Could you check a few things on this model? Use its own coordinates, in mm. Round coordinates to 2 decimals unless told otherwise and drop trailing zeros. Write each loop counter-clockwise with the first axis right and the second up, starting at its lowest first coordinate (ties: lowest second). Pieces come first, ordered by that corner, then holes. Notation, with made-up numbers: (26, 58) - (60, 58) arc R19 ccw to (60, 64) - close; hole circle Ø5 at (87, -27.5). An arc over 180 degrees is marked (long way). Put each result on its own line as item: value.
from build123d import *

# Parameters (mm, degrees)
F0_W     = 35
F0_H     = 35
F1_DEPTH = 35
F3_DEPTH = 35.001
F5_DEPTH = 35.001
F7_DEPTH = 35.001
F9_D     = 2.5
F11_D    = 2.5
F13_D    = 2.5


with BuildPart() as f1:
    # F0 (on Top) → F1 (new body)
    with BuildSketch(Plane.XY):
        with Locations((17.5, 17.5)):
            Rectangle(F0_W, F0_H)
    extrude(amount=F1_DEPTH)

    # F2 (on face) → F3 (cut, through all)
    with BuildSketch(Plane.XY.offset(35)):
        Polygon((35, 35), (0, 35), (35, 0), align=None)
    extrude(amount=-F3_DEPTH, mode=Mode.SUBTRACT)

    # F4 (on face) → F5 (cut, through all)
    with BuildSketch(Plane.XZ):
        Polygon((35, 35), (0, 0), (35, 0), align=None)
    extrude(amount=-F5_DEPTH, mode=Mode.SUBTRACT)

    # F6 (on face) → F7 (cut, through all)
    with BuildSketch(Plane(origin=(0, 0, 0), x_dir=(0, -1, 0), z_dir=(-1, 0, 0))):
        Polygon((-35, 0), (0, 0), (-35, 35), align=None)
    extrude(amount=-F7_DEPTH, mode=Mode.SUBTRACT)

    # F9 (through all)
    with Locations(Plane.XZ):
        with Locations((23, 30), (5, 12)):
            Hole(F9_D / 2)

    # F11 (through all)
    with Locations(Plane(origin=(0, 0, 0), x_dir=(0, -1, 0), z_dir=(-1, 0, 0))):
        with Locations((-23, 30), (-5, 12)):
            Hole(F11_D / 2)

    # F13 (through all)
    with Locations(Plane.XY.offset(35)):
        with Locations((5, 23), (23, 5)):
            Hole(F13_D / 2)


solid = f1.part
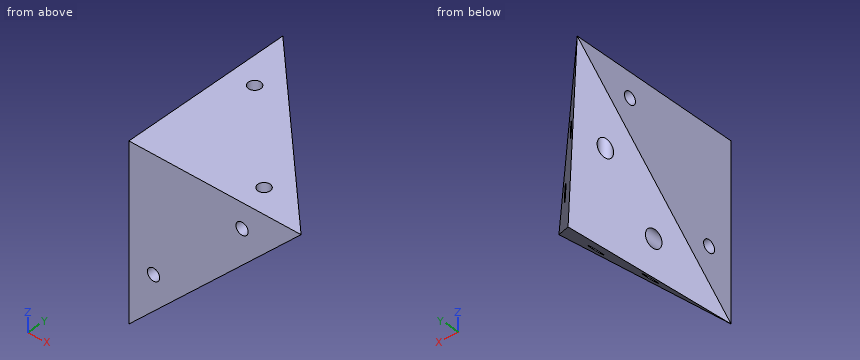
(1) Imagine slicing it at A-A, the plane y = 23. List the corners of the cut face in (x, z) for me.
Values found:
outline: (0, 23) - (3.75, 23) - (3.75, 28.75) - (0, 28.75) - close; (0, 31.25) - (3.75, 31.25) - (3.75, 35) - (0, 35) - close; (6.25, 23) - (12, 23) - (12, 28.75) - (6.25, 28.75) - close; (6.25, 31.25) - (12, 31.25) - (12, 35) - (6.25, 35) - close
(2) Imagine slicing it at B-B, the plane x = 9.5. List the corners of the cut face in (y, z) for me.
Values found:
outline: (0, 9.5) - (9.5, 9.5) - (25.5, 25.5) - (25.5, 35) - (0, 35) - close; hole circle Ø2.5 at (5, 12); hole circle Ø2.5 at (23, 30)
(3) Imagine slicing it at C-C, the plane z = 12. List the corners of the cut face in (x, y) for me.
Values found:
outline: (0, 0) - (3.75, 0) - (3.75, 3.75) - (0, 3.75) - close; (0, 6.25) - (3.75, 6.25) - (3.75, 12) - (0, 12) - close; (6.25, 0) - (12, 0) - (12, 3.75) - (6.25, 3.75) - close; (6.25, 6.25) - (12, 6.25) - (12, 12) - (6.25, 12) - close
(4) Imagine slicing it at D-D, the plane y = 11. List the corners of the cut face in (x, z) for me, then the cut area to 3 significant figures.
Values found:
outline: (0, 11) - (4.25, 11) arc R1.25 cw (long way) to (5.75, 11) - (11, 11) - (24, 24) - (24, 29.25) arc R1.25 cw (long way) to (24, 30.75) - (24, 35) - (0, 35) - close
area: 482 mm^2
(5) Please list where these lines run through material, in increasing order: probe 1 along X at (y, z) = (1, 30); probe 2 along Z at (x, y) = (5, 1.9); probe 3 along Z at (x, y) = (24, 6). Write a range as from..to.
Values found:
probe 1: x = 0..21.75, 24.25..30
probe 2: z = 5..10.75, 13.25..35
probe 3: z = 24..29.25, 30.75..35
(6) I'm going to push flat-ended pins straight in: pin 1 (12 mm diameter, centred on y = 6.5, z = 15, fed in from +X); pin 2 (5 mm diameter, centred on x = 10.5, z = 15.5, fed in from +Y); pin 3 (8 mm diameter, centred on y = 21, z = 16.5, fed in from +X). Where does each tip first touch, or does it pass through?
Values found:
pin 1: stops at x = 21
pin 2: stops at y = 18
pin 3: stops at x = 17.79
